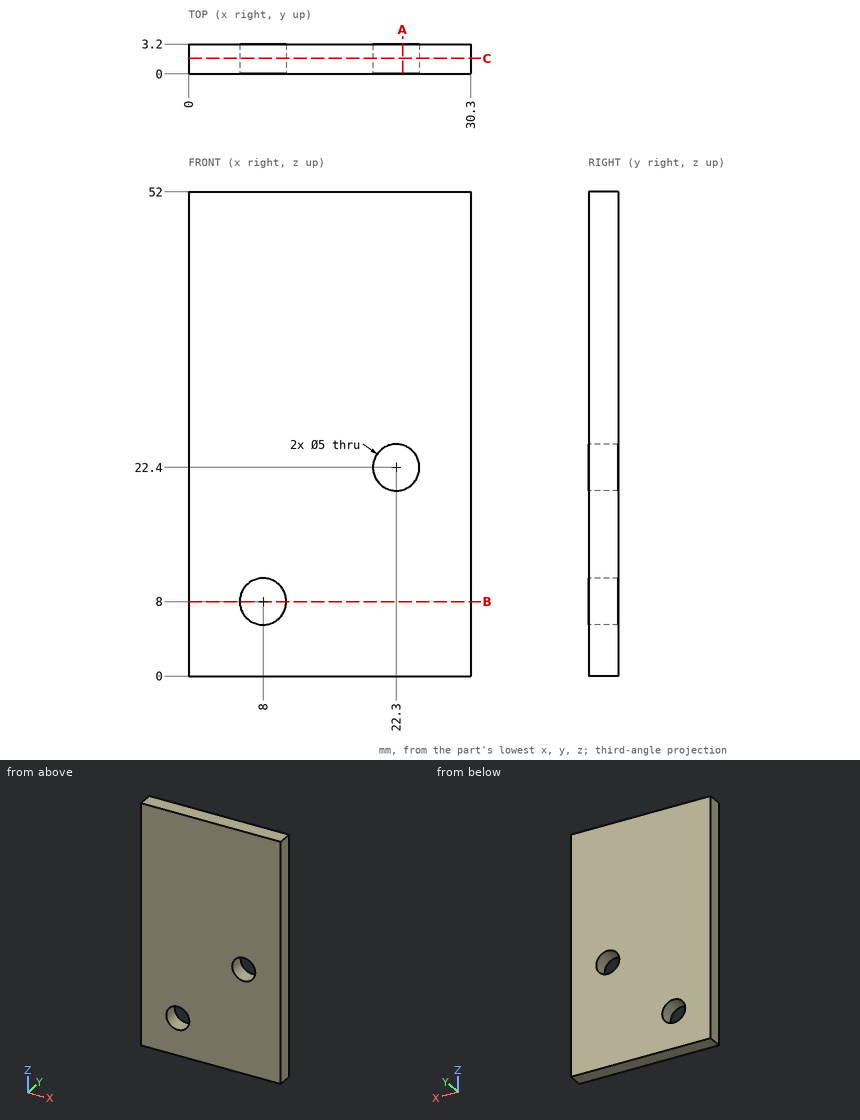
Answer from the drawing. Dimensions are ordinates in mm from the lowest x, y and z of the part. Give positions to 0.01 mm unless a question says otherwise; leave off trailing zeros. Loops run counter-clockwise (first coordinate to the right, second up) from the corner with the lowest first, then second, coordinate; pieces in that order, holes last.
Item 1: A cutting plane is placed at B-B (z = 8). Give the vertices of the cut face in (x, y).
Derived:
outline: (0, 0) - (5.5, 0) - (5.5, 3.2) - (0, 3.2) - close; (10.5, 0) - (30.3, 0) - (30.3, 3.2) - (10.5, 3.2) - close
Item 2: Find the intervals of material crossed by line 1 along Z through (x, y) = (8, 2.1); line 2 along Z through (x, y) = (22.3, 1.7); line 3 along X through (y, z) = (1.2, 8), in increasing order.
Derived:
line 1: z = 0 to 5.5, 10.5 to 52
line 2: z = 0 to 19.9, 24.9 to 52
line 3: x = 0 to 5.5, 10.5 to 30.3
Item 3: A cutting plane is placed at C-C (y = 1.65). Give the vertices of the cut face in (x, z), then the cut area to 3 significant figures.
Derived:
outline: (0, 0) - (30.3, 0) - (30.3, 52) - (0, 52) - close; hole circle Ø5 at (8, 8); hole circle Ø5 at (22.3, 22.4)
area: 1,540 mm2
Item 4: This flat-tipped pin is pushed along its axis until it touches: pin 1 Ø6.5 at (x, z) = (8, 8) entering from -Y. Where does it stop, or does it pass through?
Derived:
pin 1: stops at y = 0
Item 5: A cutting plane is placed at A-A (x = 23). Give the vertices of the cut face in (y, z), then the cut area to 3 significant figures.
Derived:
outline: (0, 0) - (3.2, 0) - (3.2, 20) - (0, 20) - close; (0, 24.8) - (3.2, 24.8) - (3.2, 52) - (0, 52) - close
area: 151 mm2
